The model under review builds one solid part; all positions refer to its coordinate system, in mm. Coordinates: 2 decimals unless noted, no trailing zeros. Order: outer loops, then holes, each group sorted by start corner. A loop starts at its lowest first (then second) coordinate and runs counter-clockwise, first axis right, second up. Notation, with made-up numbers: (18, 73) -> (53, 73) arc R18 ccw to (53, 82) -> close; hole circle Ø4 at (53.25, -0.5). An arc over 180 degrees is marked (long way). Put each result on its own line as item: value.
from build123d import *

# Parameters (mm, degrees)
SKETCH1_R           = 47.5
BOSS_EXTRUDE1_DEPTH = 6
SKETCH2_R           = 1.5
CUT_EXTRUDE1_DEPTH  = 68.44256816
SKETCH3_R           = 22.5
CUT_EXTRUDE2_DEPTH  = 68.44256816
FILLET1_R           = 3


with BuildPart() as part:
    # Sketch1 → Boss-Extrude1 (new body)
    with BuildSketch(Plane(origin=(0, 0, 0), x_dir=(1, 0, 0), z_dir=(0, 1, 0))):
        with Locations(Location((0, 0, 0), (0, 0, 270))):
            Circle(SKETCH1_R)
    extrude(amount=BOSS_EXTRUDE1_DEPTH)

    # Sketch2 → Cut-Extrude1 (cut, through all)
    with BuildSketch(Plane(origin=(0, 6, 0), x_dir=(1, 0, 0), z_dir=(0, 1, 0))):
        with Locations(Location((0, 42, 0), (0, 0, 270))):
            Circle(SKETCH2_R)
        with Locations(Location((42, 0, 0), (0, 0, 270))):
            Circle(SKETCH2_R)
        with Locations(Location((0, -42, 0), (0, 0, 270))):
            Circle(SKETCH2_R)
        with Locations(Location((-42, 0, 0), (0, 0, 270))):
            Circle(SKETCH2_R)
    extrude(amount=-CUT_EXTRUDE1_DEPTH, mode=Mode.SUBTRACT)

    # Sketch3 → Cut-Extrude2 (cut, through all)
    with BuildSketch(Plane(origin=(0, 6, 0), x_dir=(1, 0, 0), z_dir=(0, 1, 0))):
        with Locations(Location((0, 0, 0), (0, 0, 270))):
            Circle(SKETCH3_R)
    extrude(amount=-CUT_EXTRUDE2_DEPTH, mode=Mode.SUBTRACT)

    # Fillet1
    fillet1_edges = [part.edges().sort_by_distance(p)[0] for p in [
        (0, 6, -47.5),
    ]]
    fillet(fillet1_edges, radius=FILLET1_R)


solid = part.part
Item 1: For line 1 (X direction, y = 2.65, z = 0); line 2 (X direction, y = 4, z = 0); line 3 (X direction, y = 5.55, z = 15), list the stretches that pass through material, from the lowest coordinate up. Write a range as from..to.
Answers below:
line 1: -47.5..-43.5, -40.5..-22.5, 22.5..40.5, 43.5..47.5
line 2: -47.33..-43.5, -40.5..-22.5, 22.5..40.5, 43.5..47.33
line 3: -43.57..-16.77, 16.77..43.57
Item 2: Consider section C-C on y = 1.8. Write out the cut boundary in (x, z), and give its area (3 significant figures).
Answers below:
outline: circle Ø95 at (0, 0); hole circle Ø3 at (-42, 0); hole circle Ø45 at (0, 0); hole circle Ø3 at (0, -42); hole circle Ø3 at (0, 42); hole circle Ø3 at (42, 0)
area: 5,470 mm^2
Item 3: Mouldability with a two-part tool opening along X and no side actions: class faces 1 (the cylindrical face through (-46.37, 1.48, -10.3)), 2 (the flat face through (-9.9, 0, 20.4)), 3 (the cylindrical face through (-8.618, 3.042, 20.784)) as +X half, -X half, draft (parallel to the pull), parting line (faces both ways), or undercut.
Answers below:
face 1: parting line
face 2: draft
face 3: undercut
Item 4: For pin 1 Ø1.5 at (y, z) = (4, -2.5) entering from +X, flat-tipped, find the tip position at first contact; note if it passes through.
Answers below:
pin 1: x = 47.43
Item 5: Consider section B-B on z = 0. Write out the cut boundary in (x, y).
Answers below:
outline: (-47.5, 0) -> (-43.5, 0) -> (-43.5, 6) -> (-44.5, 6) arc R3 ccw to (-47.5, 3) -> close; (-40.5, 0) -> (-22.5, 0) -> (-22.5, 6) -> (-40.5, 6) -> close; (22.5, 0) -> (40.5, 0) -> (40.5, 6) -> (22.5, 6) -> close; (43.5, 0) -> (47.5, 0) -> (47.5, 3) arc R3 ccw to (44.5, 6) -> (43.5, 6) -> close
Item 6: Consider section A-A on x = 0. Write out the cut boundary in (y, z).
Answers below:
outline: (0, -47.5) -> (3, -47.5) arc R3 ccw to (6, -44.5) -> (6, -43.5) -> (0, -43.5) -> close; (0, -40.5) -> (6, -40.5) -> (6, -22.5) -> (0, -22.5) -> close; (0, 22.5) -> (6, 22.5) -> (6, 40.5) -> (0, 40.5) -> close; (0, 43.5) -> (6, 43.5) -> (6, 44.5) arc R3 ccw to (3, 47.5) -> (0, 47.5) -> close
